from build123d import *

# Parameters (mm, degrees)
BOSS_EXTRUDE1_DEPTH      = 60
BOSS_EXTRUDE2_DEPTH      = 15
BOSS_EXTRUDE3_DEPTH      = 35
BOSS_EXTRUDE3_DEPTH_BACK = 5
SKETCH1_4_R              = 15.999989418
SKETCH1_4_R_2            = 11
SKETCH2_R                = 8.5
CUT_EXTRUDE1_DEPTH       = 35


with BuildPart() as part:
    # Sketch1 → Boss-Extrude1 (new body)
    with BuildSketch(Plane.XY):
        Polygon((12.268016125, -18.108440156), (-62.731983875, -18.108440156), (-62.731983875, -36.108440156), (-7.731983875, -36.108440156), (-7.731983875, -48.108440156), (12.268016125, -48.108440156), align=None)
    extrude(amount=BOSS_EXTRUDE1_DEPTH)

    # Sketch1_3 → Boss-Extrude2 (add)
    with BuildSketch(Plane.XY):
        with BuildLine():
            Line((32.268016125, 21.891559844), (-62.731983875, -18.108440156))
            Line((-62.731983875, -18.108440156), (12.268016125, -18.108440156))
            Line((12.268016125, -18.108440156), (85.546754882, 26.199861359))
            ThreePointArc((85.546754882, 26.199861359), (64.34324961, 30.460215847), (66.754706964, 51.95263613))
            Line((66.754706964, 51.95263613), (32.268016125, 21.891559844))
        make_face()
    extrude(amount=BOSS_EXTRUDE2_DEPTH)

    # Sketch1_4 → Boss-Extrude3 (add, two sides: drawn at the far end of the back side and taken through both)
    with BuildSketch(Plane.XY.offset(-BOSS_EXTRUDE3_DEPTH_BACK)):
        with Locations((77.268019887, 39.891545268)):
            Circle(SKETCH1_4_R)
        with Locations((77.268019887, 39.891545268)):
            Circle(SKETCH1_4_R_2, mode=Mode.SUBTRACT)
    extrude(amount=BOSS_EXTRUDE3_DEPTH + BOSS_EXTRUDE3_DEPTH_BACK)

    # Sketch2 → Cut-Extrude1 (cut)
    with BuildSketch(Plane(origin=(0, -18.108440156, 0), x_dir=(1, 0, 0), z_dir=(0, 1, 0))):
        with Locations(Location((-50.731983875, -35, 0), (0, 0, 270))):
            Circle(SKETCH2_R)
        with Locations(Location((-25.731983875, -35, 0), (0, 0, 270))):
            Circle(SKETCH2_R)
    extrude(amount=-CUT_EXTRUDE1_DEPTH, mode=Mode.SUBTRACT)


solid = part.part
Verification items for the finished model (mm, model axes). A direction names the side the tool comes from. Coordinates: 2 decimals unless noted, no trailing zeros. Order: outer loops, then holes, each group sorted by start corner. A loop starts at its lowest first (then second) coordinate and runs counter-clockwise, first axis right, second up.
Item 1: Section check D-D, the plane x = -29. Enter the section's corners in (y, z), then the cut area to 3 significant figures.
Filled in:
outline: (-36.11, 0) - (-3.91, 0) - (-3.91, 15) - (-18.11, 15) - (-18.11, 27.15) - (-36.11, 27.15) - close; (-36.11, 42.85) - (-18.11, 42.85) - (-18.11, 60) - (-36.11, 60) - close
area: 1,010 mm2
Item 2: Depth check by flat-ended pin: pin 1 (13 mm diameter, centred on y = -42.5, z = 37.5, fed in from -X); pin 2 (16.5 mm diameter, centred on x = -31, z = 24.5, fed in from -Y); pin 3 (12 mm diameter, centred on y = 19.5, z = 16.5, fed in from -X); pin 4 (9 mm diameter, centred on y = -36, z = 20.5, fed in from +X). Enter the tip coordinate at first touch or a pass-through.
Filled in:
pin 1: stops at x = -62.73
pin 2: stops at y = -36.11
pin 3: stops at x = 12.79
pin 4: stops at x = 12.27
Item 3: Material ranges on L1, parallel to X at y = -22.75, z = 35; L2, parallel to X at y = -23, z = 31; L3, parallel to Y at x = -52, z = 53, recorded low to high.
Filled in:
L1: x = -62.73 to -59.23, -42.23 to -34.23, -17.23 to 12.27
L2: x = -62.73 to -58.23, -43.23 to -33.23, -18.23 to 12.27
L3: y = -36.11 to -18.11
Item 4: Access from +Z, -Z, +X, -X, +Y, -Y to the whole of each face (thin tool, end or side, straight path). Record for faces 4 (the face through (12.268, -33, 30)), 5 (the face through (-17, -30, 60)), 6 (the face through (-7.732, -42, 30)), 7 (the face through (-16, -18.108, 37)), 8 (the face through (49.75, 37.13, 7.4)).
Filled in:
face 4: +Z, -Z, +X, -Y
face 5: +Z, +X, -X, +Y, -Y
face 6: +Z, -Z, -X, -Y
face 7: +Z, +X, -X, +Y
face 8: +Z, -Z, -X, +Y
Item 5: Release check for a two-part mould opening along X. For faces 1 (the face through (-36, -36.108, 30)), 2 (the face through (48.394, 3.736, 7.395)), 3 (the face through (-44.987, -26.982, 28.735)) record: +X half, -X half, draft (parallel to the pull), parting line (faces both ways), or undercut.
Filled in:
face 1: draft
face 2: +X half
face 3: undercut
Item 6: Section check B-B, the plane y = 49. Enter the section's corners in (x, z).
Filled in:
outline: (63.37, 0) - (64.11, 0) - (64.11, -5) - (71.1, -5) - (71.1, 35) - (64.11, 35) - (64.11, 15) - (63.37, 15) - close; (83.44, -5) - (90.42, -5) - (90.42, 35) - (83.44, 35) - close
Item 7: Section check A-A, the plane z = 31. Enter the section's corners in (x, y), then the cut area to 3 significant figures.
Filled in:
outline: (-62.73, -36.11) - (-58.23, -36.11) - (-58.23, -18.11) - (-62.73, -18.11) - close; (-43.23, -36.11) - (-33.23, -36.11) - (-33.23, -18.11) - (-43.23, -18.11) - close; (-18.23, -36.11) - (-7.73, -36.11) - (-7.73, -48.11) - (12.27, -48.11) - (12.27, -18.11) - (-18.23, -18.11) - close; circle Ø32 at (77.27, 39.89); hole circle Ø22 at (77.27, 39.89)
area: 1,470 mm2
Item 8: Section check C-C, the plane z = 9.5. Enter the section's corners in (x, y), then the cut area to 3 significant figures.
Filled in:
outline: (-62.73, -36.11) - (-7.73, -36.11) - (-7.73, -48.11) - (12.27, -48.11) - (12.27, -18.11) - (85.55, 26.2) arc R16 ccw (long way) to (66.75, 51.95) - (32.27, 21.89) - (-62.73, -18.11) - close; hole circle Ø22 at (77.27, 39.89)
area: 4,910 mm2
